The model under review builds one solid part; all positions refer to its coordinate system, in mm. A direction names the side the tool comes from. Round coordinates to 2 decimals unless told otherwise and drop trailing zeros. Order: outer loops, then holes, each group sorted by start corner. A loop starts at its lowest first (then second) coordinate and runs counter-clockwise, first axis right, second up. Notation, with made-up numbers: M 30,57.5 L 47,57.5 A28 cw 47,91.5 Z; hole C 0,88.25 d8. An arc over 180 degrees is marked long. Answer as a JSON object with one key per item and string values. Group by question number.
1) The part is to be moulded in two halves that separate along X. For faces 3 (the flat face through (-3, -4, 19.05)), 4 (the cylindrical face through (-3.78, -2.9, 9.66)), 5 (the cylindrical face through (1.678, 7.555, 14.221)), say which applies: +X half, -X half, draft (parallel to the pull), parting line (faces both ways), or undercut.
2) To check wall thickness, follow line 1 (Y direction, x = 0, z = 14.5); line 2 (Y direction, x = 0, z = 7.5) (1 decimal). State the ranges of each line that lie inside material, in increasing order.
3) Insertion check: pin 1 Ø3 at (x, z) = (1, 11.5) entering from -Y; pin 2 Ø6 at (x, z) = (0.5, 13.5) entering from +Y; pin 3 Ø1 at (x, z) = (5.5, 14.5) entering from +Y; pin 4 Ø1.5 at (x, y) = (-1.5, -2) entering from +Z. Each pin has a flat end and moves straight along its axis. Give the tip position at first contact, or say it passes through.
4) Consider section D-D, the plane y = -5.75. Write out the cut boundary in (x, z) (3 decimals).
5) For faces 1 (the flat face through (0, -8, 9.525)), 2 (the flat face through (2.3, -4.4, 0)), list the 3-axis set-ups (+Z, -Z, +X, -X, +Y, -Y) from which the entire face can be reached by the end or side of a thin tool; tool diameter is ignored.
```python
from build123d import *

# Parameters (mm, degrees)
SKETCH1_R           = 9.525
BOSS_EXTRUDE1_DEPTH = 9.525
SKETCH2_R           = 7.7390625
BOSS_EXTRUDE2_DEPTH = 9.525
SKETCH3_R           = 4.7625
CUT_EXTRUDE1_DEPTH  = 24.3313898


with BuildPart() as part:
    # Sketch1 → Boss-Extrude1 (new body)
    with BuildSketch(Plane.XY):
        with Locations(Location((0, 0, 0), (0, 0, 180))):
            Circle(SKETCH1_R)
    extrude(amount=BOSS_EXTRUDE1_DEPTH)

    # Sketch2 → Boss-Extrude2 (add)
    with BuildSketch(Plane.XY.offset(9.525)):
        with Locations(Location((0, 0, 0), (0, 0, 180))):
            Circle(SKETCH2_R)
    extrude(amount=BOSS_EXTRUDE2_DEPTH)

    # Sketch3 → Cut-Extrude1 (cut, through all)
    with BuildSketch(Plane.XY.offset(19.05)):
        Circle(SKETCH3_R)
    extrude(amount=-CUT_EXTRUDE1_DEPTH, mode=Mode.SUBTRACT)


solid = part.part
```
Results list:
{
 "1": {"face 3": "draft", "face 4": "undercut", "face 5": "parting line"},
 "2": {"line 1": "-7.74 to -4.76, 4.76 to 7.74", "line 2": "-9.5 to -4.8, 4.8 to 9.5"},
 "3": {"pin 1": "y = -7.74", "pin 2": "y = 7.74", "pin 3": "y = 5.91", "pin 4": "through"},
 "4": {"outline": "M -7.594,0 L 7.594,0 L 7.594,9.525 L 5.18,9.525 L 5.18,19.05 L -5.18,19.05 L -5.18,9.525 L -7.594,9.525 Z"},
 "5": {"face 1": "+Z", "face 2": "-Z, +X, -X, +Y, -Y"}
}
